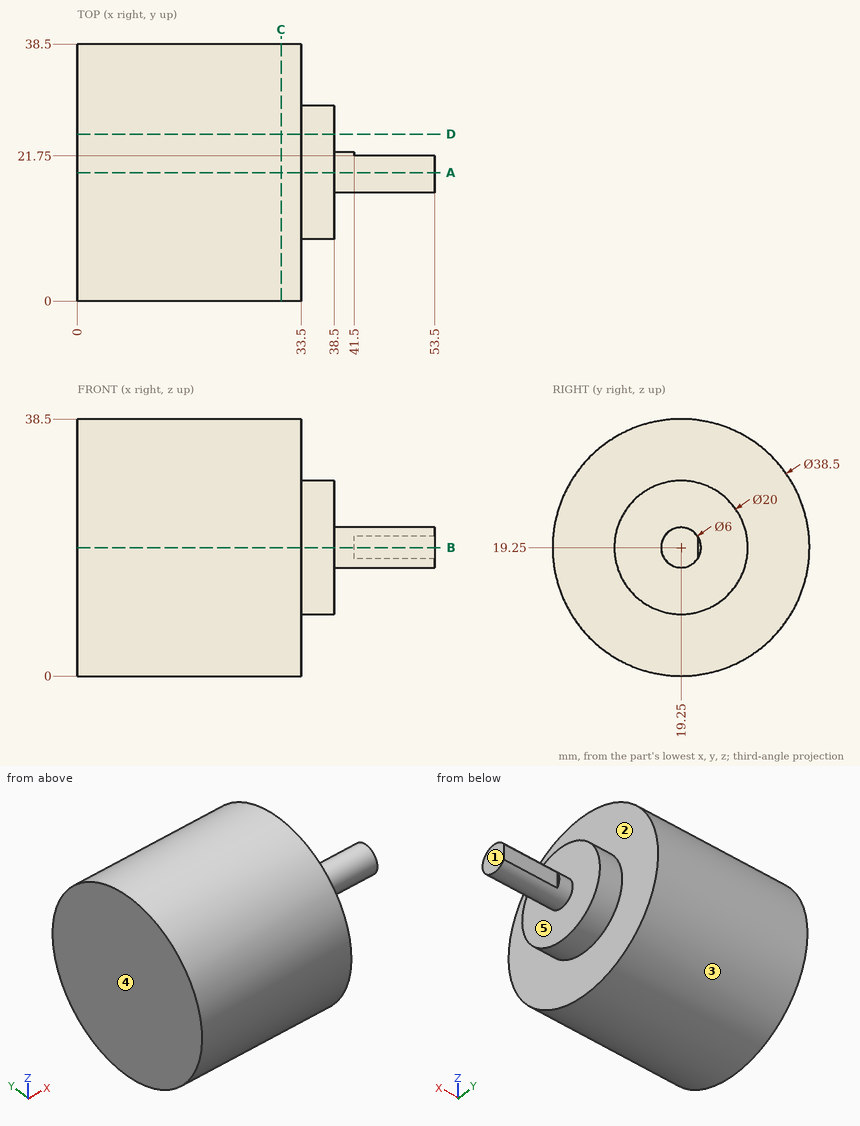
Can you work these out from the drawing? Everything is in mm from the part's minimum corner. A direction names the side the tool comes from. Round coordinates to 2 decimals unless told otherwise and drop trailing zeros. Loops run counter-clockwise (first coordinate to the right, second up) from the corner with the lowest first, then second, coordinate; pieces in that order, holes last.
1. If I drill on line 1 along X through (y, z) = (12, 12); line 2 along X through (y, z) = (19, 10); line 3 along Z through (x, y) = (8.5, 6), over which ranges is the centre line in solid material (lowest first)?
Answer list:
line 1: x = 0 to 33.5
line 2: x = 0 to 38.5
line 3: z = 5.29 to 33.21
2. For P1, Ø8, axis at x = 6.5, y = 26.5, coming from the -Z side; P2, Ø2, axis at x = 9, y = 5.5, coming from the +Z side; P3, Ø5, axis at x = 22, y = 8, coming from the -Z side; P4, Ø10, axis at y = 21.5, z = 12.5, coming from the -X side, each with a flat end and sliding along its axis, tell me the tip position at first contact or that it passes through.
Answer list:
P1: stops at z = 0.28
P2: stops at z = 33.67
P3: stops at z = 2.1
P4: stops at x = 0
3. If we section it at C-C on x = 30.5: Write out the boundary of the cut face in (y, z), plus the area to 3 significant figures.
Answer list:
outline: circle Ø38.5 at (19.25, 19.25)
area: 1,160 mm2
4. If we section it at A-A on y = 19.25: Write out the boundary of the cut face in (x, z).
Answer list:
outline: (0, 0) - (33.5, 0) - (33.5, 9.25) - (38.5, 9.25) - (38.5, 16.25) - (53.5, 16.25) - (53.5, 22.25) - (38.5, 22.25) - (38.5, 29.25) - (33.5, 29.25) - (33.5, 38.5) - (0, 38.5) - close
5. If we section it at D-D on y = 25: Write out the boundary of the cut face in (x, z).
Answer list:
outline: (0, 0.88) - (33.5, 0.88) - (33.5, 11.07) - (38.5, 11.07) - (38.5, 27.43) - (33.5, 27.43) - (33.5, 37.62) - (0, 37.62) - close
6. If we section it at B-B on z = 19.25: Write out the boundary of the cut face in (x, y).
Answer list:
outline: (0, 0) - (33.5, 0) - (33.5, 9.25) - (38.5, 9.25) - (38.5, 16.25) - (53.5, 16.25) - (53.5, 21.75) - (41.5, 21.75) - (41.5, 22.25) - (38.5, 22.25) - (38.5, 29.25) - (33.5, 29.25) - (33.5, 38.5) - (0, 38.5) - close
7. Which directions (+Z, -Z, +X, -X, +Y, -Y) give clear straight access to the entire face, cutting with the end or side of a thin tool? Please do the marked faces 1 and 2.
Answer list:
face 1: +Z, -Z, +X, +Y, -Y
face 2: +X
8. We'd pull the mould along X, two halves only. Please class the marked faces 3, 4 and 5: +X half, -X half, draft (parallel to the pull), parting line (faces both ways), or undercut.
Answer list:
face 3: draft
face 4: -X half
face 5: +X half
